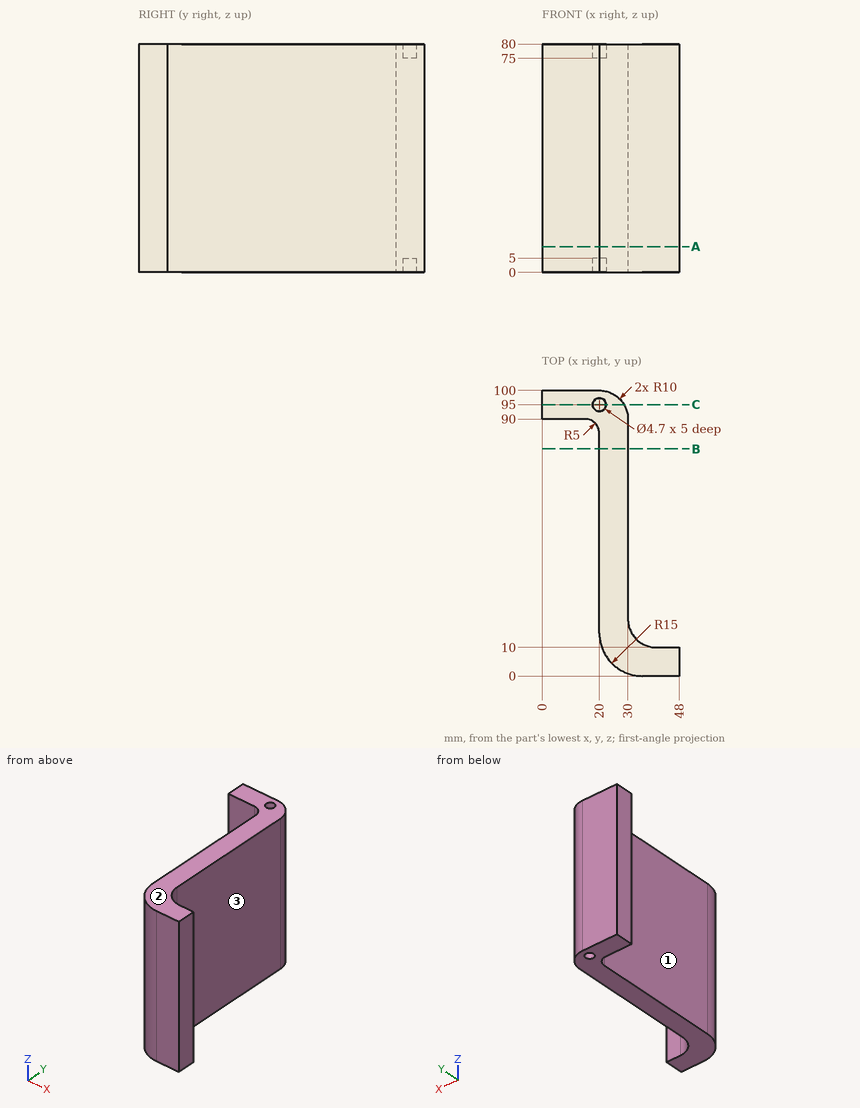
Study the drawing (mm; zero at the part's minimum x, y, z) and answer. A direction names the side the tool comes from. Give positions to 0.01 mm unless a question says otherwise; leave off trailing zeros. Write each loop counter-clockwise with the first axis right and the second up, starting at its lowest first coordinate (ties: lowest second). Pieces come first, ordered by that corner, then holes. Notation, with made-up numbers: (87, -5.75) -> (136, -5.75) arc R23 ccw to (136, 6.25) -> close; hole circle Ø8 at (19.25, 46). An arc over 180 degrees is marked (long way). Answer in a Markdown table with one row per item.
1) Section B-B on y = 79.5 is taken. Give the vertices of the cut face in (x, z).
Results list:
| item | result |
|---|---|
| outline | (20, 0) -> (30, 0) -> (30, 80) -> (20, 80) -> close |
2) Section A-A on z = 9 is taken. Give the vertices of the cut face in (x, y).
Results list:
| item | result |
|---|---|
| outline | (0, 90) -> (15, 90) arc R5 cw to (20, 85) -> (20, 15) arc R15 ccw to (35, 0) -> (48, 0) -> (48, 10) -> (40, 10) arc R10 cw to (30, 20) -> (30, 90) arc R10 ccw to (20, 100) -> (0, 100) -> close |
3) Each of these flat-tipped pins is pushed along its axis until it touches: pin 1 Ø12 at (x, z) = (7, 25.5) entering from -Y; pin 2 Ø9 at (x, z) = (44, 53.5) entering from +Y; pin 3 Ø2 at (x, z) = (28, 19.5) entering from +Y; pin 4 Ø3 at (x, y) = (32.5, 78.5) entering from +Z. Where does it stop, or does it pass through?
Results list:
| item | result |
|---|---|
| pin 1 | y = 90 |
| pin 2 | y = 10.01 |
| pin 3 | y = 97.14 |
| pin 4 | through |
4) A tool of negligible diameter and unlimited length cuts with its end or side. For the marked faces 1, 2 and 3, from which of +Z, -Z, +X, -X, +Y, -Y can it reach the whole face along a straight path? Write none if from no direction.
Results list:
| item | result |
|---|---|
| face 1 | +Z, -Z, -X, -Y |
| face 2 | +Z, +X, -X, +Y, -Y |
| face 3 | +Z, -Z, +X, +Y |
5) Section C-C on y = 95 is taken. Give the vertices of the cut face in (x, z), plus the area to 3 significant figures.
Results list:
| item | result |
|---|---|
| outline | (0, 0) -> (17.65, 0) -> (17.65, 5) -> (22.35, 5) -> (22.35, 0) -> (28.66, 0) -> (28.66, 80) -> (22.35, 80) -> (22.35, 75) -> (17.65, 75) -> (17.65, 80) -> (0, 80) -> close |
| area | 2,250 mm^2 |
6) Straight lines are drawn through the part: line 1 (X direction, y = 74, z = 25.5); line 2 (Y direction, x = 13, z = 69); line 3 (X direction, y = 95, z = 2). For each, find the intervals that lie inside material, in ascending order. Write a range as [from, to].
Results list:
| item | result |
|---|---|
| line 1 | [20, 30] |
| line 2 | [90, 100] |
| line 3 | [0, 17.65], [22.35, 28.66] |
